Part print with two shaded views. Sizes in mm from the minimum x, y, z corner. A direction names the side the tool comes from. Give positions to 0.01 mm unless a question says otherwise; leave off trailing zeros. Write each loop counter-clockwise with the first axis right and the second up, starting at its lowest first coordinate (ties: lowest second). Pieces come first, ordered by that corner, then holes. Notation, with made-up numbers: (86.5, -8.75) - (139.5, -8.75) arc R17 ccw to (139.5, 19.25) - close; hole circle Ø4 at (68, 71). An arc over 180 degrees is marked (long way). One line per item, written item: value. Start each with the question number.
(1) Probe L1, parallel to Y at x = 3.75, z = 4.5; L2, parallel to Y at x = 5, z = 6.5; L3, parallel to Y at x = 4, z = 2.5. List the from-to ranges inside material, lowest first.
(2) Drop flat-ended pins along their axis: P1, Ø3, axis at y = 8.5, z = 9, coming from the -X side; P2, Ø2, axis at y = 3, z = 3.5, coming from the +X side; P3, Ø1.5, axis at y = 8, z = 10.5, coming from the +X side. Give the stop position or say it passes through.
(3) Cut at A-A, the plane x = 6.5. List the corners of the cut face in (y, z).
(4) 3-axis set-ups, long thin cutter, end or side, ignore diameter. For the marked faces 1 and 2: which of +Z, -Z, +X, -X, +Y, -Y reach the whole face in a straight line?
(5) Cut at C-C, the plane x = 9.5. List the corners of the cut face in (y, z), and give its area (3 significant figures).
(6) Cut at B-B, the plane z = 6.5. List the corners of the cut face in (x, y), and give its area (4 significant figures).
(7) Cut at D-D, the plane y = 14. List the corners of the cut face in (x, z), and give its area (3 significant figures).
(8) Mould opens along Y. For the marked faces 3, 4 and 5 say: pulls with the +Y half, pulls with the -Y half, needs draft (parallel to the pull), parting line crosses it, or undercut.
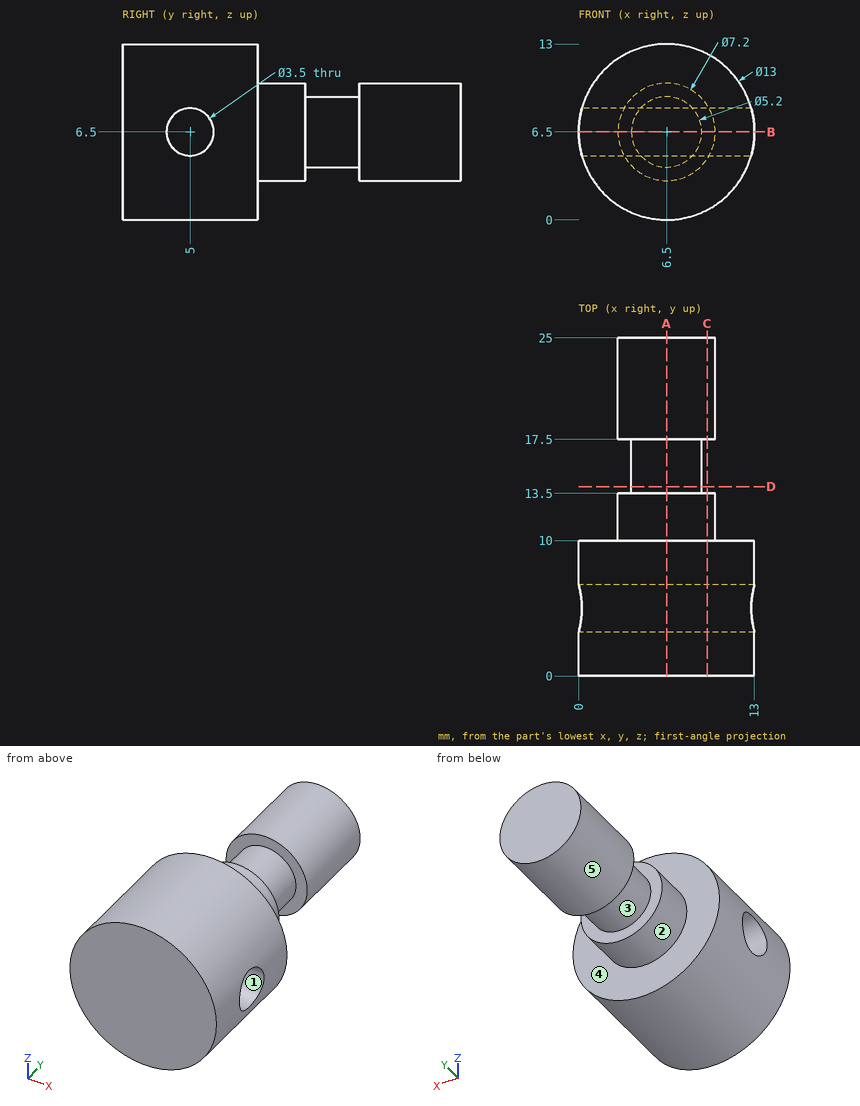
Answers follow:
1. L1: y = 0 to 13.5, 17.5 to 25
1. L2: y = 0 to 3.25, 6.75 to 25
1. L3: y = 0 to 10
2. P1: stops at x = 0.08
2. P2: stops at x = 12.68
2. P3: stops at x = 12.13
3. outline: (0, 0) - (10, 0) - (10, 2.9) - (13.5, 2.9) - (13.5, 3.9) - (17.5, 3.9) - (17.5, 2.9) - (25, 2.9) - (25, 10.1) - (17.5, 10.1) - (17.5, 9.1) - (13.5, 9.1) - (13.5, 10.1) - (10, 10.1) - (10, 13) - (0, 13) - close; hole circle Ø3.5 at (5, 6.5)
4. face 1: +X, -X
4. face 2: +Y
5. outline: (0, 0.73) - (10, 0.73) - (10, 4.51) - (13.5, 4.51) - (13.5, 8.49) - (10, 8.49) - (10, 12.27) - (0, 12.27) - close; (17.5, 4.51) - (25, 4.51) - (25, 8.49) - (17.5, 8.49) - close; hole circle Ø3.5 at (5, 6.5)
5. area: 149 mm²
6. outline: (0, 0) - (13, 0) - (13, 3.25) - (0, 3.25) - close; (0, 6.75) - (13, 6.75) - (13, 10) - (10.1, 10) - (10.1, 13.5) - (9.1, 13.5) - (9.1, 17.5) - (10.1, 17.5) - (10.1, 25) - (2.9, 25) - (2.9, 17.5) - (3.9, 17.5) - (3.9, 13.5) - (2.9, 13.5) - (2.9, 10) - (0, 10) - close
6. area: 184.5 mm²
7. outline: circle Ø5.2 at (6.5, 6.5)
7. area: 21.2 mm²
8. face 3: undercut
8. face 4: pulls with the +Y half
8. face 5: needs draft
